Verification items for the finished model (mm, model axes). Face numbers are marked on the shaded views. A direction names the side the tool comes from. Give positions to 0.01 mm unless a question says otherwise; leave off trailing zeros. Loops run counter-clockwise (first coordinate to the right, second up) from the corner with the lowest first, then second, coordinate; pieces in that order, holes last. Notation, with made-up numbers: (88.25, 70) - (96.25, 70) arc R19 ccw to (96.25, 85) - close; hole circle Ø1 at (80.25, 72). An arc over 180 degrees is marked (long way). Answer in a Markdown table with one row per item.
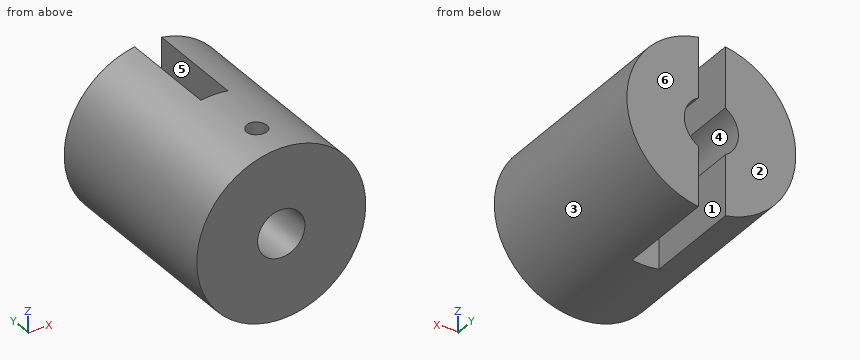
```python
from build123d import *

# Parameters (mm, degrees)
CROQUIS1_R              = 12.5
SALIENTE_EXTRUIR1_DEPTH = 30
CORTAR_EXTRUIR1_DEPTH   = 15
CROQUIS3_R              = 3.5
CORTAR_EXTRUIR2_DEPTH   = 15
CROQUIS4_R              = 1.5
CORTAR_EXTRUIR3_DEPTH   = 15


with BuildPart() as part:
    # Croquis1 → Saliente-Extruir1 (new body)
    with BuildSketch(Plane(origin=(0, 0, 0), x_dir=(1, 0, 0), z_dir=(0, 1, 0))):
        with Locations(Location((0, 0, 0), (0, 0, 270))):
            Circle(CROQUIS1_R)
    extrude(amount=SALIENTE_EXTRUIR1_DEPTH)

    # Croquis2 → Cortar-Extruir1 (cut)
    with BuildSketch(Plane(origin=(0, 30, 0), x_dir=(1, 0, 0), z_dir=(0, 1, 0))):
        with BuildLine():
            Line((-2.073774887, 3.420447006), (-2.073774887, 12.856138783))
            Line((-2.073774887, 12.856138783), (1.926225113, 12.856138783))
            Line((1.926225113, 12.856138783), (1.926225113, 3.505660681))
            ThreePointArc((1.926225113, 3.505660681), (4, 0), (1.926225113, -3.505660681))
            Line((1.926225113, -3.505660681), (1.926225113, -12.772374377))
            Line((1.926225113, -12.772374377), (-2.073774887, -12.772374377))
            Line((-2.073774887, -12.772374377), (-2.073774887, -3.420447006))
            ThreePointArc((-2.073774887, -3.420447006), (-4, 0), (-2.073774887, 3.420447006))
        make_face()
    extrude(amount=-CORTAR_EXTRUIR1_DEPTH, mode=Mode.SUBTRACT)

    # Croquis3 → Cortar-Extruir2 (cut)
    with BuildSketch(Plane.XZ):
        with Locations(Location((0, 0, 0), (0, 0, 270))):
            Circle(CROQUIS3_R)
    extrude(amount=-CORTAR_EXTRUIR2_DEPTH, mode=Mode.SUBTRACT)

    # Croquis4 → Cortar-Extruir3 (cut)
    with BuildSketch(Plane.XY.offset(15)):
        with Locations((0, 5.510659623)):
            Circle(CROQUIS4_R)
    extrude(amount=-CORTAR_EXTRUIR3_DEPTH, mode=Mode.SUBTRACT)


solid = part.part
```
Q1. Draft check along X on the marked faces 1, 2 and 3. Enter one of: +X half, -X half, draft (parallel to the pull), parting line (faces both ways), or undercut.
Completed:
| item | result |
|---|---|
| face 1 | undercut |
| face 2 | draft |
| face 3 | parting line |
Q2. Tool access check on the marked faces 4, 5 and 6. Record the directions out of +Z, -Z, +X, -X, +Y, -Y that give a thin tool (end or side, any length) a straight path to the whole face; none if there is none.
Completed:
| item | result |
|---|---|
| face 4 | +Y |
| face 5 | +Z, -Z, +Y |
| face 6 | +Z, -Z, +X, -X, +Y |
Q3. Sectioned sample at C-C (z = 0). Record the cut outline in (x, y).
Completed:
| item | result |
|---|---|
| outline | (-12.5, 0) - (-3.5, 0) - (-3.5, 15) - (-4, 15) - (-4, 30) - (-12.5, 30) - close; (3.5, 0) - (12.5, 0) - (12.5, 30) - (4, 30) - (4, 15) - (3.5, 15) - close |
Q4. Thickness scan on line 1 (Z direction, x = 0, y = 11); line 2 (Y direction, x = 0, z = 7.5); line 3 (X direction, y = 9, z = 0.25). Record the ranges inside material, lowest first.
Completed:
| item | result |
|---|---|
| line 1 | -12.5 to -3.5, 3.5 to 12.5 |
| line 2 | 0 to 4.01, 7.01 to 15 |
| line 3 | -12.5 to -3.49, 3.49 to 12.5 |
Q5. Go/stop test with flat-tipped pins: P1, Ø8, axis at y = 23, z = -4.5, coming from the +X side; P2, Ø12, axis at x = -7, y = 17, coming from the +Z side; P3, Ø7, axis at y = 24, z = 10, coming from the +X side; P4, Ø1.5, axis at x = -0.5, y = 24.5, coming from the -Z side. Record where each tip stops, or that it passes through.
Completed:
| item | result |
|---|---|
| P1 | x = 12.49 |
| P2 | z = 12.43 |
| P3 | x = 10.68 |
| P4 | through |
Q6. Sectioned sample at D-D (z = 9.5). Record the cut outline in (x, y).
Completed:
| item | result |
|---|---|
| outline | (-8.12, 0) - (8.12, 0) - (8.12, 30) - (1.93, 30) - (1.93, 15) - (-2.07, 15) - (-2.07, 30) - (-8.12, 30) - close; hole circle Ø3 at (0, 5.51) |
Q7. Sectioned sample at B-B (y = 19.5). Record the cut outline in (x, z).
Completed:
| item | result |
|---|---|
| outline | (-2.07, -12.33) - (-2.07, -3.42) arc R4 cw to (-2.07, 3.42) - (-2.07, 12.33) arc R12.5 ccw to start; (1.93, -12.35) arc R12.5 ccw to (1.93, 12.35) - (1.93, 3.51) arc R4 cw to (1.93, -3.51) - close |
Q8. Sectioned sample at A-A (x = 0). Record the cut outline in (y, z), and give its area (3 significant figures).
Completed:
| item | result |
|---|---|
| outline | (0, -12.5) - (15, -12.5) - (15, -3.5) - (0, -3.5) - close; (0, 3.5) - (4.01, 3.5) - (4.01, 12.5) - (0, 12.5) - close; (7.01, 3.5) - (15, 3.5) - (15, 12.5) - (7.01, 12.5) - close |
| area | 243 mm^2 |
